```python
from build123d import *

# Parameters (mm, degrees)
BOSS_EXTRUDE2_DEPTH     = 10
ESQUISSE2_W             = 255
ESQUISSE2_H             = 170
ESQUISSE2_W_2           = 234
ESQUISSE2_H_2           = 149.5
ENL_V_MAT_EXTRU_1_DEPTH = 1
ENL_V_MAT_EXTRU_2_DEPTH = 1
CONG_1_R                = 10
CONG_2_R                = 10
CONG_3_R                = 5
CONG_4_R                = 5
ESQUISSE5_R             = 2
ENL_V_MAT_EXTRU_3_DEPTH = 2
ESQUISSE6_R             = 2.05
ENL_V_MAT_EXTRU_4_DEPTH = 10
ESQUISSE7_R             = 2.05
ENL_V_MAT_EXTRU_5_DEPTH = 10


with BuildPart() as part:
    # Sketch1 → Boss-Extrude2 (new body)
    with BuildSketch(Plane.XY):
        Polygon((-200, 0), (200, 0), (200, 170), (200, 256.402135463), (127.5, 170), (-127.5, 170), (-200, 256.402135463), (-200, 170), align=None)
    extrude(amount=BOSS_EXTRUDE2_DEPTH)

    # Esquisse2 → Enlèv. mat.-Extru.1 (cut)
    with BuildSketch(Plane.XY.offset(10)):
        with Locations((0, 85)):
            Rectangle(ESQUISSE2_W, ESQUISSE2_H)
        with Locations((0, 85.25)):
            Rectangle(ESQUISSE2_W_2, ESQUISSE2_H_2, mode=Mode.SUBTRACT)
    extrude(amount=-ENL_V_MAT_EXTRU_1_DEPTH, mode=Mode.SUBTRACT)

    # Esquisse3 → Enlèv. mat.-Extru.2 (cut)
    with BuildSketch(Plane.XY.offset(10)):
        Polygon((127.5, 170), (135.160444431, 163.572123903), (200, 240.844897194), (200, 256.402135463), align=None)
        Polygon((-200, 256.402135463), (-127.5, 170), (-135.160444431, 163.572123903), (-200, 240.844897194), align=None)
    extrude(amount=-ENL_V_MAT_EXTRU_2_DEPTH, mode=Mode.SUBTRACT)

    # Congé1
    cong_1_edges = [part.edges().sort_by_distance(p)[0] for p in [
        (200, 0, 5),
    ]]
    fillet(cong_1_edges, radius=CONG_1_R)

    # Congé2
    cong_2_edges = [part.edges().sort_by_distance(p)[0] for p in [
        (-200, 0, 5),
    ]]
    fillet(cong_2_edges, radius=CONG_2_R)

    # Congé3
    cong_3_edges = [part.edges().sort_by_distance(p)[0] for p in [
        (-200, 256.402135463, 4.5),
    ]]
    fillet(cong_3_edges, radius=CONG_3_R)

    # Congé4
    cong_4_edges = [part.edges().sort_by_distance(p)[0] for p in [
        (200, 256.402135463, 4.5),
    ]]
    fillet(cong_4_edges, radius=CONG_4_R)

    # Esquisse5 → Enlèv. mat.-Extru.3 (cut)
    with BuildSketch(Plane.XY.offset(10)):
        with Locations((-135.160444431, 163.572123903)):
            Circle(ESQUISSE5_R)
        with Locations(Location((135.160444431, 163.572123903, 0), (0, 0, 50))):
            Circle(ESQUISSE5_R)
    extrude(amount=-ENL_V_MAT_EXTRU_3_DEPTH, mode=Mode.SUBTRACT)

    # Esquisse6 → Enlèv. mat.-Extru.4 (cut)
    with BuildSketch(Plane(origin=(0, 0, 0), x_dir=(-1, 0, 0), z_dir=(0, 0, -1))):
        with Locations((-70.5, 165)):
            Circle(ESQUISSE6_R)
        with Locations((-122.5, 135)):
            Circle(ESQUISSE6_R)
        with Locations(Location((122.5, 135, 0), (0, 0, 180))):
            Circle(ESQUISSE6_R)
        with Locations(Location((70.5, 165, 0), (0, 0, 180))):
            Circle(ESQUISSE6_R)
        with Locations((70.5, 5)):
            Circle(ESQUISSE6_R)
        with Locations((122.5, 35)):
            Circle(ESQUISSE6_R)
        with Locations(Location((-122.5, 35, 0), (0, 0, 180))):
            Circle(ESQUISSE6_R)
        with Locations(Location((-70.5, 5, 0), (0, 0, 180))):
            Circle(ESQUISSE6_R)
    extrude(amount=-ENL_V_MAT_EXTRU_4_DEPTH, mode=Mode.SUBTRACT)

    # Esquisse7 → Enlèv. mat.-Extru.5 (cut)
    with BuildSketch(Plane(origin=(0, 0, 0), x_dir=(-1, 0, 0), z_dir=(0, 0, -1))):
        with Locations((143.777848565, 181.620565373)):
            Circle(ESQUISSE7_R)
        with Locations(Location((181.870852493, 227.018039657, 0), (0, 0, 180))):
            Circle(ESQUISSE7_R)
        with Locations((-181.870852493, 227.018039657)):
            Circle(ESQUISSE7_R)
        with Locations(Location((-143.777848565, 181.620565373, 0), (0, 0, 180))):
            Circle(ESQUISSE7_R)
    extrude(amount=-ENL_V_MAT_EXTRU_5_DEPTH, mode=Mode.SUBTRACT)


solid = part.part
```
Work out the finished part from the listing and answer in its coordinate system (mm). A direction names the side the tool comes from. Round coordinates to 2 decimals unless told otherwise and drop trailing zeros. Write each loop counter-clockwise with the first axis right and the second up, starting at its lowest first coordinate (ties: lowest second). Pieces come first, ordered by that corner, then holes.
1) Which of the six approach directions +Z, -Z, +X, -X, +Y, -Y give full straight-line access (tool end or side, diameter ignored) to faces 1 (the face through (159.78, 208.47, 4.44)), 2 (the face through (167.778, 202.444, 9.507)), 3 (the face through (-2, 86, 10))?
2) Flat-ended cylindrical pins translate along their axes: P1, Ø4.5, axis at x = 181.87, y = 227.02, coming from the +Z side; P2, Ø2.5, axis at x = -135.16, y = 163.57, coming from the +Z side; P3, Ø4.5, axis at x = 135.16, y = 163.57, coming from the -Z side; P4, Ø0.5, axis at x = -24, z = 9.5, coming from the -Y side. Find the tip coordinate at first contact, or state that the pin passes through.
3) A cutting plane is placed at A-A on x = -16. Determine the outline of the cut face in (y, z), and give its area (3 significant figures).
4) Consider probe 1 along X at (y, z) = (165, 6.75); probe 2 along Y at (x, z) = (70.5, 4.5); probe 3 along X at (y, z) = (135, 2.5). Determine where each line is inside the solid, lowest interval first.
5) Determine the mould class of faces 4 (the face through (164, 206, 9)), 5 (the face through (196.99, 2.85, 5.07)), 6 (the face through (-3, 98, 0)), 7 (the face through (-200, 128, 5)) for opening direction X: pulls with the +X half, pulls with the -X half, needs draft (parallel to the pull), parting line crosses it, or undercut.
6) A cutting plane is placed at C-C on z = 1.75. Give the number of separate pieces and of enclosed holes in the cut face, and give its area (3 significant figures).
7) A cutting plane is placed at B-B on y = 194. Determine the outline of the cut face in (x, z), and give its area (3 significant figures).
Entries:
1. face 1: +Z, -Z, +Y
1. face 2: +Z, +Y
1. face 3: +Z, +X, -X, +Y, -Y
2. P1: stops at z = 9
2. P2: stops at z = 8
2. P3: stops at z = 0
2. P4: stops at y = 10.5
3. outline: (0, 0) - (170, 0) - (170, 9) - (160, 9) - (160, 10) - (10.5, 10) - (10.5, 9) - (0, 9) - close
3. area: 1,680 mm2
4. probe 1: x = -200 to -72.55, -68.45 to 68.45, 72.55 to 200
4. probe 2: y = 0 to 2.95, 7.05 to 162.95, 167.05 to 170
4. probe 3: x = -200 to -124.55, -120.45 to 120.45, 124.55 to 200
5. face 4: undercut
5. face 5: pulls with the +X half
5. face 6: needs draft
5. face 7: pulls with the -X half
6. separate pieces: 1
6. enclosed holes: 12
6. area: 74,000 mm2
7. outline: (-200, 0) - (-147.64, 0) - (-147.64, 9) - (-160.69, 9) - (-160.69, 10) - (-200, 10) - close; (147.64, 0) - (200, 0) - (200, 10) - (160.69, 10) - (160.69, 9) - (147.64, 9) - close
7. area: 1,020 mm2
